Work out the finished part from the listing and answer in its coordinate system (mm). A direction names the side the tool comes from. Coordinates: 2 decimals unless noted, no trailing zeros. Order: outer loops, then holes, each group sorted by start corner. A loop starts at its lowest first (then second) coordinate and runs counter-clockwise, first axis right, second up. Notation, with made-up numbers: (-0.5, 4.25) -> (21.5, 4.25) arc R19 cw to (21.5, 27.25) -> close; hole circle Ø7 at (-22, 64.5). An arc over 180 degrees is marked (long way). Write item = value, one per line. Start each with the question number.
Q1. Flat-ended cylindrical pins translate along their axes: pin 1 (14.5 mm diameter, centred on y = 191, z = 82, fed in from +X); pin 2 (5.5 mm diameter, centred on y = 414, z = 121, fed in from -X); pin 3 (3 mm diameter, centred on x = -234, y = 528.5, fed in from +Z). Find the tip coordinate at first contact, or state that the pin passes through.
Q2. The part is cut by section A-A, the plane x = 196. Determine the outline of the cut face in (y, z).
Q3. Which of the six approach directions +Z, -Z, +X, -X, +Y, -Y give full straight-line access (tool end or side, diameter ignored) to faces 1 (the flat face through (215, -232, 230)), 2 (the flat face through (171, 185.851, 87)), 3 (the flat face through (-182, 689.851, 87)), 4 (the flat face through (-85.69, 928.98, 87.02))?
Q4. The part is cut by section B-B, the plane y = -92. Determine the outline of the cut face in (x, z).
Q5. For a pull along X with two mould halves and no side action, classify faces 5 (the flat face through (-39.473, 56.219, 87.02)), 6 (the flat face through (-167, 403.851, 87)), 7 (the flat face through (39.473, 492.219, 87.02)), 8 (the flat face through (42.31, 469.6, 87.02)) as +X half, -X half, draft (parallel to the pull), parting line (faces both ways), or undercut.
Q6. The part is cut by section C-C, the plane z = 350.5. Determine the outline of the cut face in (x, y).
Q7. The part is cut by section D-D, the plane y = 1457.5. Determine the outline of the cut face in (x, z).
Q8. Straight lines are drawn through the part: L1, parallel to Y at x = -185, z = 105; L2, parallel to Y at x = -120.5, z = 79; L3, parallel to Y at x = 188.5, z = 272.5. For each, find the intervals that lie inside material, in ascending order. Write a range as from..to.
```python
from build123d import *

# Parameters (mm, degrees)
F0_W     = 590
F0_H     = 2170
F1_DEPTH = 18
F3_DEPTH = 140
F4_W     = 430
F4_H     = 430
F5_DEPTH = 430


with BuildPart() as f1:
    # F0 (on Top) → F1 (new body)
    with BuildSketch(Plane.XY):
        with Locations((0.711598, 640.850716)):
            Rectangle(F0_W, F0_H)
    extrude(amount=F1_DEPTH)

    # F2 (on face) → F3 (join)
    with BuildSketch(Plane.XY.offset(18)):
        Polygon((-9, 25.74664), (-9, -444.149284), (9, -444.149284), (9, 118.290795), (9, 143.74664), (9, 436.290795), (9, 461.74664), (9, 701.140038), (9, 726.595882), (9, 926.713631), (9, 952.169475), (9, 1255.850716), (-9, 1255.850716), (-9, 852.287224), (-9, 826.83138), (-9, 591.240543), (-9, 565.784699), (-9, 369.202484), (-9, 343.74664), (-9, 51.202484), align=None)
        Polygon((-69.104076, 85.850716), (-9, 25.74664), (-9, 51.202484), (-61.648232, 103.850716), (-261.648232, 103.850716), (-261.648232, 85.850716), align=None)
        Polygon((9, 143.74664), (9, 118.290795), (76.559921, 185.850716), (269.104076, 185.850716), (269.104076, 203.850716), (69.104076, 203.850716), align=None)
        Polygon((-69.104076, 403.850716), (-9, 343.74664), (-9, 369.202484), (-61.648232, 421.850716), (-261.648232, 421.850716), (-261.648232, 403.850716), align=None)
        Polygon((9, 461.74664), (9, 436.290795), (76.559921, 503.850716), (269.104076, 503.850716), (269.104076, 521.850716), (69.104076, 521.850716), align=None)
        Polygon((-115.066017, 671.850716), (-9, 565.784699), (-9, 591.240543), (-107.610173, 689.850716), (-257.610173, 689.850716), (-257.610173, 671.850716), align=None)
        Polygon((9, 726.595882), (9, 701.140038), (79.710678, 771.850716), (222.254834, 771.850716), (222.254834, 789.850716), (72.254834, 789.850716), align=None)
        Polygon((-172.019336, 989.850716), (-9, 826.83138), (-9, 852.287224), (-164.563492, 1007.850716), (-264.563492, 1007.850716), (-264.563492, 989.850716), align=None)
        Polygon((9, 952.169475), (9, 926.713631), (122.137085, 1039.850716), (214.681241, 1039.850716), (214.681241, 1057.850716), (114.681241, 1057.850716), align=None)
    extrude(amount=F3_DEPTH)

    # F4 (on face) → F5 (join)
    with BuildSketch(Plane.XY.offset(18)):
        with Locations((0, -229.149284)):
            Rectangle(F4_W, F4_H)
    extrude(amount=F5_DEPTH)


solid = f1.part
```
Model answer:
q1.pin_1 = 269.1
q1.pin_2 = -261.65
q1.pin_3 = 18
q2.outline = (-444.15, 0) -> (1725.85, 0) -> (1725.85, 18) -> (1057.85, 18) -> (1057.85, 158) -> (1039.85, 158) -> (1039.85, 18) -> (789.85, 18) -> (789.85, 158) -> (771.85, 158) -> (771.85, 18) -> (521.85, 18) -> (521.85, 158) -> (503.85, 158) -> (503.85, 18) -> (203.85, 18) -> (203.85, 158) -> (185.85, 158) -> (185.85, 18) -> (-14.15, 18) -> (-14.15, 448) -> (-444.15, 448) -> close
q3.face_1 = +Z, +X, -Y
q3.face_2 = +Z, +X
q3.face_3 = +Z, -X
q3.face_4 = +Z, +Y
q4.outline = (-294.29, 0) -> (295.71, 0) -> (295.71, 18) -> (215, 18) -> (215, 448) -> (-215, 448) -> (-215, 18) -> (-294.29, 18) -> close
q5.face_5 = -X half
q5.face_6 = draft
q5.face_7 = undercut
q5.face_8 = +X half
q6.outline = (-215, -444.15) -> (215, -444.15) -> (215, -14.15) -> (-215, -14.15) -> close
q7.outline = (-294.29, 0) -> (295.71, 0) -> (295.71, 18) -> (-294.29, 18) -> close
q8.L1 = -444.15..-14.15, 85.85..103.85, 403.85..421.85, 671.85..689.85, 989.85..1007.85
q8.L2 = -444.15..-14.15, 85.85..103.85, 403.85..421.85, 671.85..689.85, 938.33..963.79
q8.L3 = -444.15..-14.15
